Here's how the part is built. I have some questions about the finished solid (model axes, mm). A direction names the side the tool comes from. Coordinates: 2 decimals unless noted, no trailing zeros. Order: outer loops, then holes, each group sorted by start corner. A loop starts at its lowest first (then second) coordinate and runs counter-clockwise, first axis right, second up. Notation, with made-up numbers: (11.5, 5) - (40.5, 5) arc R22 cw to (40.5, 34) - close; hole circle Ø10 at (31, -23). An arc over 180 degrees is marked (long way). Answer as CSV lines item,"result". Start each with the question number.
Q1. Suppose I cut it at A-A (y = -8). Please give me the cut outline in (x, z).
Q2. For faces 5 (the face through (34, -6, -26)), 6 (the face through (-33, -10, 26.7)), 7 (the face through (24, -6, -30.5)), 8 (the face through (14, -6, -26)), 9 (the face through (24, -6, -21.5)), which set-ups out of +Z, -Z, +X, -X, +Y, -Y let a thin tool reach every point of the face, with its end or its side?
Q3. Thinking about a two-plate mould opening in Z: for faces 1 (the face through (36, -21, 2)), 2 (the face through (44.785, 0.789, -28.364)), 3 (the face through (-33, -10, -23.3)), 4 (the face through (-48.7, -10, 1)), which applies, released by +Z, released by -Z, zero draft, split by the parting line, or undercut?
Q4. Suppose I cut it at C-C (z = 30). Please give me the cut outline in (x, y).
Q5. Suppose I cut it at B-B (x = 45). Please give me the cut outline in (y, z), then the cut area to 3 significant figures.
Q6. Suppose I cut it at D-D (z = -11.5). Please give me the cut outline in (x, y).
Q7. For pin 1 Ø10 at (x, y) = (34, -13) entering from -Z; pin 2 Ø8 at (x, z) = (-23.5, 19.5) entering from -Y; pin 3 Ø4 at (x, z) = (45, -30) entering from -Y, each with a flat end and sliding along its axis, tell me the tip position at first contact or that it passes through.
Q8. I need wall thicknesses on line 1 (Z direction, x = 45, y = 0.9); line 2 (X direction, y = -13, z = 26); line 3 (Y direction, x = -11, z = 17). Which ranges of each line are inside material? Lowest first, please.
from build123d import *

# Parameters (mm, degrees)
F0_W     = 100
F0_H     = 70
F0_R     = 1.65
F0_W_2   = 20
F0_H_2   = 9
F0_W_3   = 32
F0_H_3   = 50
F0_R_2   = 3
F1_DEPTH = 1.6
F2_DEPTH = 20.2
F3_DEPTH = 12.5
F4_DEPTH = 42


with BuildPart() as f1:
    # F0 (on Front) → F1 (new body)
    with BuildSketch(Plane.XZ):
        Rectangle(F0_W, F0_H)
        with Locations((-45, -30)):
            Circle(F0_R, mode=Mode.SUBTRACT)
        with Locations((24, -26)):
            Rectangle(F0_W_2, F0_H_2, mode=Mode.SUBTRACT)
        with Locations((45, -30)):
            Circle(F0_R, mode=Mode.SUBTRACT)
        with Locations((-32.7, 1.7)):
            Rectangle(F0_W_3, F0_H_3, mode=Mode.SUBTRACT)
        with Locations((-45, 30)):
            Circle(F0_R, mode=Mode.SUBTRACT)
        with Locations((39, 2)):
            Circle(F0_R_2, mode=Mode.SUBTRACT)
        with Locations((45, 30)):
            Circle(F0_R, mode=Mode.SUBTRACT)
        with Locations((-32.7, 1.7)):
            Rectangle(F0_W_3, F0_H_3)
        with Locations((24, -26)):
            Rectangle(F0_W_2, F0_H_2)
        with Locations((39, 2)):
            Circle(F0_R_2)
    extrude(amount=-F1_DEPTH)

    # F0 (on Front) → F2 (join)
    with BuildSketch(Plane.XZ):
        with Locations((-32.7, 1.7)):
            Rectangle(F0_W_3, F0_H_3)
    extrude(amount=F2_DEPTH)

    # F0 (on Front) → F3 (join)
    with BuildSketch(Plane.XZ):
        with Locations((24, -26)):
            Rectangle(F0_W_2, F0_H_2)
    extrude(amount=F3_DEPTH)

    # F0 (on Front) → F4 (join)
    with BuildSketch(Plane.XZ):
        with Locations((39, 2)):
            Circle(F0_R_2)
    extrude(amount=F4_DEPTH)


solid = f1.part
Here are the results:
1,outline,"(-48.7, -23.3) - (-16.7, -23.3) - (-16.7, 26.7) - (-48.7, 26.7) - close; (14, -30.5) - (34, -30.5) - (34, -21.5) - (14, -21.5) - close; circle Ø6 at (39, 2)"
2,face 5,"+Z, -Z, +X, -Y"
2,face 6,"+Z, +X, -X, -Y"
2,face 7,"-Z, +X, -X, -Y"
2,face 8,"+Z, -Z, -Y"
2,face 9,"+Z, +X, -Y"
3,face 1,"split by the parting line"
3,face 2,"undercut"
3,face 3,"released by -Z"
3,face 4,"zero draft"
4,outline,"(-50, 0) - (-46.65, 0) - (-46.65, 1.6) - (-50, 1.6) - close; (-43.35, 0) - (43.35, 0) - (43.35, 1.6) - (-43.35, 1.6) - close; (46.65, 0) - (50, 0) - (50, 1.6) - (46.65, 1.6) - close"
5,outline,"(0, -35) - (1.6, -35) - (1.6, -31.65) - (0, -31.65) - close; (0, -28.35) - (1.6, -28.35) - (1.6, 28.35) - (0, 28.35) - close; (0, 31.65) - (1.6, 31.65) - (1.6, 35) - (0, 35) - close"
5,area,"101 mm²"
6,outline,"(-50, 0) - (-48.7, 0) - (-48.7, -20.2) - (-16.7, -20.2) - (-16.7, 0) - (50, 0) - (50, 1.6) - (-50, 1.6) - close"
7,pin 1,"stops at z = -30.5"
7,pin 2,"stops at y = -20.2"
7,pin 3,"stops at y = 0"
8,line 1,"z = -35 to -31.65, -28.35 to 28.35, 31.65 to 35"
8,line 2,"x = -48.7 to -16.7"
8,line 3,"y = 0 to 1.6"
